```python
from build123d import *

# Parameters (mm, degrees)
F1_DEPTH    = 53
F2_W        = 9.7
F2_H        = 17
F3_DEPTH    = 7
F4_R        = 1.95
F5_DEPTH    = 25
F6_T1_DEPTH = 42
F7_R        = 1.95
F8_DEPTH    = 7


# Not quite as in the source:
# - a fillet or chamfer that OpenCascade refuses, or shapes differently, is made with other operations: its cross-section is extruded or revolved along the edge and cut away or added
# - a pattern or mirror of a feature is missing from the dataset's text; its kind, count and spacing are read off the source's solid


with BuildPart() as f1:
    # F0 (on Right) → F1 (new body, symmetric)
    with BuildSketch(Plane.YZ):
        Polygon((-17.2, 0), (0, 0), (0, -15), (2, -15), (2, 2), (-19.2, 2), (-19.2, -5), (-17.2, -5), align=None)
    extrude(amount=F1_DEPTH, both=True)

    # F2 (on face) → F3 (join)
    with BuildSketch(Plane(origin=(0, 2, 0), x_dir=(-1, 0, 0), z_dir=(0, 1, 0))):
        with Locations((-48.15, -6.5)):
            Rectangle(F2_W, F2_H)
    f3 = extrude(amount=F3_DEPTH)

    # F3_copies: F3 across plane
    add(f3.mirror(Plane(origin=(0, 0, 0), x_dir=(0, 0, -1), z_dir=(-1, 0, 0))))

    # F4 (on face) → F5 (cut)
    with BuildSketch(Plane.XY.offset(2)):
        with Locations((48.15, 5)):
            Circle(F4_R)
    f5 = extrude(amount=-F5_DEPTH, mode=Mode.SUBTRACT)

    # F5_copies: F5 across plane
    add(f5.mirror(Plane(origin=(0, 0, 0), x_dir=(0, 0, -1), z_dir=(-1, 0, 0))), mode=Mode.SUBTRACT)

    # F6: fillet of radius 5 on 4 edges, made by hand

    # F6_s2 → F6_t1 (cut)
    with BuildSketch(Plane.XY.offset(-27.5)):
        with BuildLine():
            ThreePointArc((53, 4), (51.5355339059, 7.5355339059), (48, 9))
            Line((48, 9), (53, 9))
            Line((53, 9), (53, 4))
        make_face()
        with BuildLine():
            ThreePointArc((48.3, 9), (44.7644660941, 7.5355339059), (43.3, 4))
            Line((43.3, 4), (43.3, 9))
            Line((43.3, 9), (48.3, 9))
        make_face()
        with BuildLine():
            ThreePointArc((-53, 4), (-51.5355339059, 7.5355339059), (-48, 9))
            Line((-48, 9), (-53, 9))
            Line((-53, 9), (-53, 4))
        make_face()
        with BuildLine():
            ThreePointArc((-48.3, 9), (-44.7644660941, 7.5355339059), (-43.3, 4))
            Line((-43.3, 4), (-43.3, 9))
            Line((-43.3, 9), (-48.3, 9))
        make_face()
    extrude(amount=F6_T1_DEPTH, mode=Mode.SUBTRACT)

    # F7 (on face) → F8 (join)
    with BuildSketch(Plane(origin=(0, 0, -15), x_dir=(1, 0, 0), z_dir=(0, 0, -1))):
        with Locations((48.15, -5)):
            Circle(F7_R)
    f8 = extrude(amount=-F8_DEPTH)

    # F8_copies: F8 across plane
    add(f8.mirror(Plane(origin=(0, 0, 0), x_dir=(0, 0, -1), z_dir=(-1, 0, 0))))


solid = f1.part
```
The model under review builds one solid part; all positions refer to its coordinate system, in mm. A direction names the side the tool comes from. Coordinates: 2 decimals unless noted, no trailing zeros. Order: outer loops, then holes, each group sorted by start corner. A loop starts at its lowest first (then second) coordinate and runs counter-clockwise, first axis right, second up. Notation, with made-up numbers: (25, -7.5) -> (54, -7.5) arc R25 cw to (54, 22.5) -> close; hole circle Ø4 at (39, -35). An arc over 180 degrees is marked (long way). Answer in a Markdown table with one row per item. Add a question column.
Item 1: We need section D-D on y = -14.5. Write out the cut boundary in (x, z).
Item 2: Mouldability with a two-part tool opening along Y and no side actions: class faces 5 (the cylindrical face through (-44.75, 7.52, -6.62)), 6 (the flat face through (48, 5, -8)), 7 (the flat face through (1, 0, -7)), 8 (the flat face through (1, -19.2, -1)) as +Y half, -Y half, draft (parallel to the pull), parting line (faces both ways), or undercut.
Item 3: We need section A-A on z = -11.25. Write out the cut boundary in (x, y).
Item 4: We need section B-B on x = -36. Write out the cut boundary in (y, z), plus the area to 3 significant figures.
Item 5: Machinability: for faces 1 (the flat face through (1, -18, -5)), 2 (the flat face through (43.3, 3, -7)), 3 (the flat face through (1, -17.2, -3)), 4 (the cylindrical face through (-49.95, 4.25, -2.93)), which of the approach directions +Z, -Z, +X, -X, +Y, -Y give a long, thin tool a straight path to every point of the face, cutting with its end or side? Answer none if there is none.
Item 6: Clearance check with flat-ended pins moving along their axes: pin 1 (0.6 mm diameter, centred on x = 5.5, y = -18, fed in from -Z); pin 2 (2 mm diameter, centred on x = 48, y = 5, fed in from +Z); pin 3 (5 mm diameter, centred on x = 17.5, z = -13, fed in from +Y); pin 4 (2 mm diameter, centred on y = 5, z = -11, fed in from -X). State where each tip first meets the part, or that it passes through.
Item 7: We need section C-C on y = 5. Write out the cut boundary in (x, z).
Item 8: To check wall thickness, follow probe 1 along Y at (x, z) = (-48.15, -1.5); probe 2 along Y at (x, z) = (-35, -3.75); probe 3 along X at (y, z) = (5, -0.75). State the ranges of each line that lie inside material, in increasing order.
Final values:
| question | item | result |
|---|---|---|
| 1 | outline | (-53, 0) -> (53, 0) -> (53, 2) -> (-53, 2) -> close |
| 2 | face 5 | +Y half |
| 2 | face 6 | undercut |
| 2 | face 7 | undercut |
| 2 | face 8 | -Y half |
| 3 | outline | (-53, 0) -> (53, 0) -> (53, 4) arc R5 ccw to (48.15, 9) arc R5 ccw to (43.3, 4) -> (43.3, 2) -> (-43.3, 2) -> (-43.3, 4) arc R5 ccw to (-48.15, 9) arc R5 ccw to (-53, 4) -> close |
| 4 | outline | (-19.2, -5) -> (-17.2, -5) -> (-17.2, 0) -> (0, 0) -> (0, -15) -> (2, -15) -> (2, 2) -> (-19.2, 2) -> close |
| 4 | area | 82.4 mm2 |
| 5 | face 1 | -Z, +X, -X, -Y |
| 5 | face 2 | +Z, -Z, +Y |
| 5 | face 3 | -Z, +X, -X |
| 5 | face 4 | +Z |
| 6 | pin 1 | stops at z = -5 |
| 6 | pin 2 | stops at z = -8 |
| 6 | pin 3 | stops at y = 2 |
| 6 | pin 4 | stops at x = -53 |
| 7 | outline | (-52.9, -15) -> (-43.4, -15) -> (-43.4, 2) -> (-46.2, 2) -> (-46.2, -8) -> (-50.1, -8) -> (-50.1, 2) -> (-52.9, 2) -> close; (43.4, -15) -> (52.9, -15) -> (52.9, 2) -> (50.1, 2) -> (50.1, -8) -> (46.2, -8) -> (46.2, 2) -> (43.4, 2) -> close |
| 8 | probe 1 | y = -19.2 to -17.2, 0 to 3.05, 6.95 to 9 |
| 8 | probe 2 | y = -19.2 to -17.2, 0 to 2 |
| 8 | probe 3 | x = -52.9 to -50.1, -46.2 to -43.4, 43.4 to 46.2, 50.1 to 52.9 |
